from build123d import *

# Parameters (mm, degrees)
BOSS_EXTRUDE1_DEPTH = 1.5
SKETCH2_R           = 3.25
SKETCH2_R_2         = 1
SKETCH2_R_3         = 1.5
CUT_EXTRUDE1_DEPTH  = 20


with BuildPart() as part:
    # Sketch1 → Boss-Extrude1 (new, symmetric)
    with BuildSketch(Plane.XY):
        with BuildLine():
            Line((0, -4.75), (262, -4.75))
            Line((262, -4.75), (262, 4.75))
            Line((262, 4.75), (0, 4.75))
            ThreePointArc((0, 4.75), (-4.75, 0), (0, -4.75))
        make_face()
    extrude(amount=BOSS_EXTRUDE1_DEPTH, both=True)

    # Sketch2 → Cut-Extrude1 (cut, symmetric)
    with BuildSketch(Plane.XY):
        Circle(SKETCH2_R)
        with Locations((127, 0)):
            Circle(SKETCH2_R_2)
        with Locations((254, 0)):
            Circle(SKETCH2_R_3)
    extrude(amount=CUT_EXTRUDE1_DEPTH, both=True, mode=Mode.SUBTRACT)


solid = part.part
The model under review builds one solid part; all positions refer to its coordinate system, in mm. Coordinates: 2 decimals unless noted, no trailing zeros. Loops run counter-clockwise (first coordinate to the right, second up) from the corner with the lowest first, then second, coordinate; pieces in that order, holes last.
(1) Wall thickness on L1, parallel to Y at x = 127, z = 0.4; L2, parallel to Y at x = 0, z = 0.6; L3, parallel to X at y = 0.75, z = 0.4: over which ranges is each line inside the solid? List them lowest first.
Determined:
L1: y = -4.75 to -1, 1 to 4.75
L2: y = -4.75 to -3.25, 3.25 to 4.75
L3: x = -4.69 to -3.16, 3.16 to 126.34, 127.66 to 252.7, 255.3 to 262
(2) Draft analysis for pull direction Y (two halves, no side actions). For faces 1 (the flat face through (127, 2, 1.5)), 2 (the cylindrical face through (-4.75, 0.1, 0.02)), 3 (the cylindrical face through (-2.579, -1.978, 0.021)), state which applies: +Y half, -Y half, draft (parallel to the pull), parting line (faces both ways), or undercut.
Determined:
face 1: draft
face 2: parting line
face 3: undercut
(3) Consider section A-A, the plane z = 0.8. Give the boundary of the cut face in (x, y).
Determined:
outline: (0, -4.75) - (262, -4.75) - (262, 4.75) - (0, 4.75) arc R4.75 ccw to start; hole circle Ø6.5 at (0, 0); hole circle Ø2 at (127, 0); hole circle Ø3 at (254, 0)
